from build123d import *

# Parameters (mm, degrees)
SKETCH1_R                   = 35
BOSS_EXTRUDE1_DEPTH         = 10
SKETCH2_R                   = 23
BOSS_EXTRUDE2_DEPTH         = 7
BOSS_EXTRUDE3_DEPTH         = 4
SKETCH4_R                   = 1.5
CUT_EXTRUDE2_DEPTH          = 4
SKETCH5_W                   = 2
SKETCH5_H                   = 6
BOSS_EXTRUDE4_DEPTH         = 10
FILLET1_RADIUS              = 1
FILLET1_LENGTH              = 10
FILLET2_R                   = 2
FILLET1_OF_MIRROR2_2_RADIUS = 1
FILLET1_OF_MIRROR2_2_LENGTH = 10
FILLET2_OF_MIRROR2_R        = 2
SKETCH6_R                   = 15
CUT_EXTRUDE3_DEPTH          = 10


with BuildPart() as part:
    # Sketch1 → Boss-Extrude1 (new body)
    with BuildSketch(Plane.YZ):
        with Locations(Location((0, 0, 0), (0, 0, 270))):
            Circle(SKETCH1_R)
    extrude(amount=BOSS_EXTRUDE1_DEPTH)

    # Sketch2 → Boss-Extrude2 (add)
    with BuildSketch(Plane.YZ.offset(10)):
        with Locations(Location((0, 0, 0), (0, 0, 270))):
            Circle(SKETCH2_R)
    extrude(amount=BOSS_EXTRUDE2_DEPTH)

    # Sketch3 → Boss-Extrude3 (add)
    with BuildSketch(Plane(origin=(0, 0, 13), x_dir=(0, 1, 0), z_dir=(0, 0, 1))):
        Polygon((35, -17), (-35, -17), (-45.711191774, -25.987757067), (-45.711191774, -30.987757067), (-23, -50.044709708), (23, -50.044709708), (45.711191774, -30.987757067), (45.711191774, -25.987757067), align=None)
    boss_extrude3 = extrude(amount=-BOSS_EXTRUDE3_DEPTH)

    # Sketch4 → Cut-Extrude2 (cut)
    with BuildSketch(Plane.XY.offset(13)):
        with Locations((28.487757067, -42.711191774)):
            Circle(SKETCH4_R)
        with Locations(Location((28.487757067, 42.711191774, 0), (0, 0, 180))):
            Circle(SKETCH4_R)
    cut_extrude2 = extrude(amount=-CUT_EXTRUDE2_DEPTH, mode=Mode.SUBTRACT)

    # Sketch5 → Boss-Extrude4 (add)
    with BuildSketch(Plane.YZ.offset(17)):
        with Locations((0, 16)):
            Rectangle(SKETCH5_W, SKETCH5_H)
    boss_extrude4 = extrude(amount=BOSS_EXTRUDE4_DEPTH)

    # Fillet1: full round fillet: the end face becomes a half cylinder, R = half its width
    fillet1_face = Plane((22, 0, 19), x_dir=(-1, 0, 0), z_dir=(0, 0, 1))  # on the end face: x along it, z out of the body
    fillet1_slab = fillet1_face.offset(-FILLET1_RADIUS / 2) * Box(FILLET1_LENGTH, 2 * FILLET1_RADIUS, FILLET1_RADIUS, mode=Mode.PRIVATE)  # the body's end, R deep
    fillet1_round = Plane((22, 0, 18), x_dir=(0, 0, 1), z_dir=(-1, 0, 0)) * Cylinder(FILLET1_RADIUS, FILLET1_LENGTH, mode=Mode.PRIVATE)  # its axis R under the face
    add(fillet1_slab - fillet1_round, mode=Mode.SUBTRACT)

    # Fillet2
    fillet2_edges = [part.edges().sort_by_distance(p)[0] for p in [
        (50.044709708, 23, 11),
        (50.044709708, -23, 11),
        (30.987757067, -45.711191774, 11),
        (25.987757067, -45.711191774, 11),
        (17, -35, 11),
        (17, 35, 11),
        (25.987757067, 45.711191774, 11),
        (30.987757067, 45.711191774, 11),
    ]]
    fillet(fillet2_edges, radius=FILLET2_R)

    # Mirror2: Boss-Extrude3, Cut-Extrude2, Boss-Extrude4 across plane
    add(boss_extrude3.mirror(Plane.XY))
    add(cut_extrude2.mirror(Plane.XY), mode=Mode.SUBTRACT)
    add(boss_extrude4.mirror(Plane.XY))

    # Fillet1 of Mirror2 2: full round fillet: the end face becomes a half cylinder, R = half its width
    fillet1_of_mirror2_2_face = Plane((22, 0, -19), x_dir=(-1, 0, 0), z_dir=(0, 0, -1))  # on the end face: x along it, z out of the body
    fillet1_of_mirror2_2_slab = fillet1_of_mirror2_2_face.offset(-FILLET1_OF_MIRROR2_2_RADIUS / 2) * Box(FILLET1_OF_MIRROR2_2_LENGTH, 2 * FILLET1_OF_MIRROR2_2_RADIUS, FILLET1_OF_MIRROR2_2_RADIUS, mode=Mode.PRIVATE)  # the body's end, R deep
    fillet1_of_mirror2_2_round = Plane((22, 0, -18), x_dir=(0, 0, -1), z_dir=(-1, 0, 0)) * Cylinder(FILLET1_OF_MIRROR2_2_RADIUS, FILLET1_OF_MIRROR2_2_LENGTH, mode=Mode.PRIVATE)  # its axis R under the face
    add(fillet1_of_mirror2_2_slab - fillet1_of_mirror2_2_round, mode=Mode.SUBTRACT)

    # Fillet2 of Mirror2
    fillet2_of_mirror2_edges = [part.edges().sort_by_distance(p)[0] for p in [
        (50.044709708, 23, -11),
        (50.044709708, -23, -11),
        (30.987757067, -45.711191774, -11),
        (25.987757067, -45.711191774, -11),
        (17, -35, -11),
        (17, 35, -11),
        (25.987757067, 45.711191774, -11),
        (30.987757067, 45.711191774, -11),
    ]]
    fillet(fillet2_of_mirror2_edges, radius=FILLET2_OF_MIRROR2_R)

    # Sketch6 → Cut-Extrude3 (cut)
    with BuildSketch(Plane(origin=(0, 0, 0), x_dir=(0, -1, 0), z_dir=(-1, 0, 0))):
        with Locations(Location((0, 0, 0), (0, 0, 90))):
            Circle(SKETCH6_R)
    extrude(amount=-CUT_EXTRUDE3_DEPTH, mode=Mode.SUBTRACT)


solid = part.part
Design review of the part built by this model. Coordinates are the model's own, in mm. A direction names the side the tool comes from. Round coordinates to 2 decimals unless told otherwise and drop trailing zeros. Loops run counter-clockwise (first coordinate to the right, second up) from the corner with the lowest first, then second, coordinate; pieces in that order, holes last. Notation, with made-up numbers: (55, 33) -> (82, 33) arc R18 cw to (82, 52) -> close; hole circle Ø3 at (-26, 41). An arc over 180 degrees is marked (long way). Use one line per item in the form item = value. Start each with the question number.
Q1. Draft analysis for pull direction Z (two halves, no side actions). For faces 6 (the face through (27, 0, 16)), 7 (the face through (17, 0, 0)), state which applies: +Z half, -Z half, draft (parallel to the pull), parting line (faces both ways), or undercut.
Q2. Wall thickness on line 1 along Z through (x, y) = (46, -19.5); line 2 along X through (y, z) = (24, 22); line 3 along Y through (x, z) = (20, -15): over which ranges is each line inside the solid? List them lowest first. Write a range as [from, to].
Q3. We need section A-A on z = 0. Give the boundary of the cut face in (x, y).
Q4. For pin 1 Ø10 at (x, y) = (28.5, 4) entering from -Z; pin 2 Ø3 at (x, y) = (27.5, -13) entering from -Z; pin 3 Ø4 at (y, z) = (6, -24) entering from +X; pin 4 Ø2.5 at (x, y) = (28.49, 42.71) entering from -Z, all flat-tipped, find the tip position at first contact; note any pin that passes through.
Q5. We need section C-C on y = -27.5. Give the boundary of the cut face in (x, z).
Q6. We need section B-B on x = 33. Give the boundary of the cut face in (y, z).
Q7. Machinability: for faces 1 (the face through (27, 0, -16)), 2 (the face through (22, 1, 15)), 3 (the face through (22, -1, -15)), 4 (the face through (22, -1, 15)), 5 (the face through (17, 0, -20)), which of the approach directions +Z, -Z, +X, -X, +Y, -Y give a long, thin tool a straight path to every point of the face, cutting with its end or side? Answer none if there is none.
Q8. We need section D-D on x = 7.5. Give the boundary of the cut face in (y, z), then the cut area to 3 significant figures.
Calculated:
q1.face_6 = draft
q1.face_7 = undercut
q2.line_1 = [-13, -9], [9, 13]
q2.line_2 = [0, 10]
q2.line_3 = [-1, 1]
q3.outline = (0, -35) -> (10, -35) -> (10, -23) -> (17, -23) -> (17, 23) -> (10, 23) -> (10, 35) -> (0, 35) -> (0, 15) -> (10, 15) -> (10, -15) -> (0, -15) -> close
q4.pin_1 = -19
q4.pin_2 = -13
q4.pin_3 = 17
q4.pin_4 = through
q5.outline = (0, -21.65) -> (10, -21.65) -> (10, 21.65) -> (0, 21.65) -> close; (17, -13) -> (46.27, -13) -> (46.27, -9) -> (17, -9) -> close; (17, 9) -> (46.27, 9) -> (46.27, 13) -> (17, 13) -> close
q6.outline = (-43.31, -13) -> (43.31, -13) -> (43.31, -9) -> (-43.31, -9) -> close; (-43.31, 9) -> (43.31, 9) -> (43.31, 13) -> (-43.31, 13) -> close
q7.face_1 = -Z, +X, +Y, -Y
q7.face_2 = +Z, +X, +Y
q7.face_3 = -Z, +X, -Y
q7.face_4 = +Z, +X, -Y
q7.face_5 = -Z, +X
q8.outline = circle Ø70 at (0, 0); hole circle Ø30 at (0, 0)
q8.area = 3,140 mm²
